Input: dimensioned drawing with shaded views. Units: mm. Origin: part minimum x, y, z. Give positions to 0.01 mm unless a question says otherwise; leave off trailing zeros. Write each loop counter-clockwise with the first axis right and the second up, starting at its lowest first coordinate (ties: lowest second). Pieces come first, ordered by that corner, then holes. Notation, with made-up numbers: (-14, 6) -> (45, 6) arc R11 ccw to (45, 18) -> close; hole circle Ø2 at (37.5, 21.5). An arc over 180 degrees is marked (long way). Return JSON: item names as keys, results as strings. Group by question number.
Item 1: Section B-B, the plane y = 72. Return loops of the section in (x, z).
Item 2: Section A-A, the plane x = 63.5. Return loops of the section in (y, z).
Item 3: Section C-C, the plane z = 3. Count the separate pieces of the cut face and the enclosed holes in it.
Item 4: Pin query (flat end, axial travel): P1, Ø1.9, axis at x = 32, z = 4, coming from the +Y side; P2, Ø3, axis at x = 124.5, z = 4.5, coming from the +Y side; P3, Ø3, axis at y = 92, z = 2, coming from the +X side. Return the tip coordinate at first contact, or that it passes through.
Item 5: Line query: line 1 (Y direction, x = 6, z = 1); line 2 (X direction, y = 86.5, z = 3.25); line 3 (X direction, y = 19, z = 1.75). Output: solid intervals per line, ascending. Write a range as [from, to].
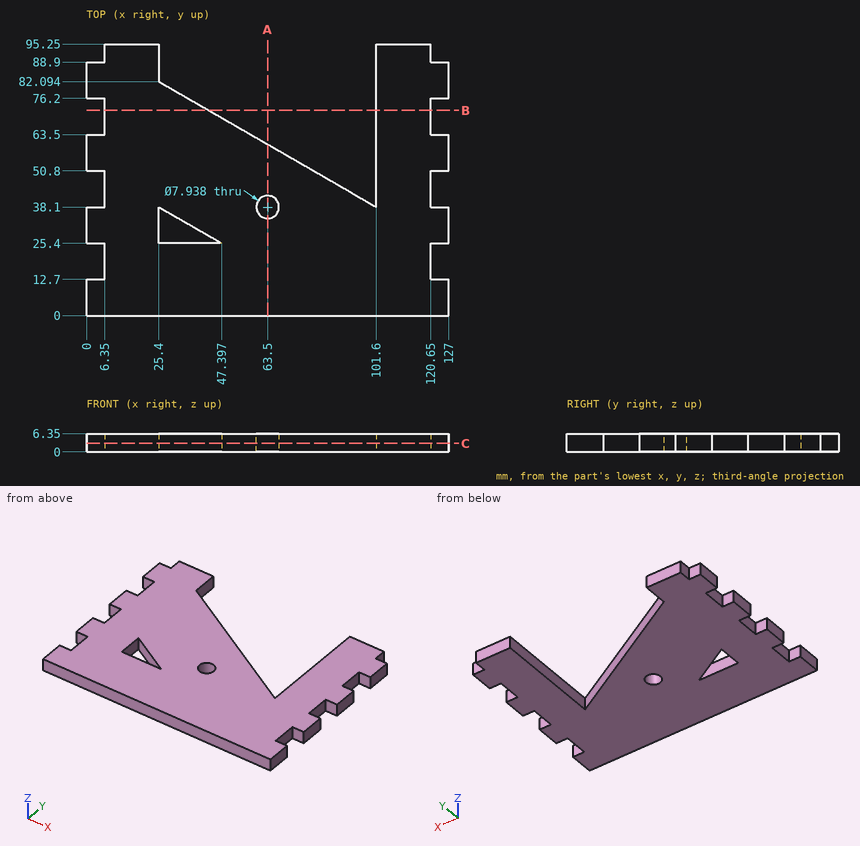
Answer below:
{
 "1": {"outline": "(6.35, 0) -> (42.88, 0) -> (42.88, 6.35) -> (6.35, 6.35) -> close; (101.6, 0) -> (120.65, 0) -> (120.65, 6.35) -> (101.6, 6.35) -> close"},
 "2": {"outline": "(0, 0) -> (34.13, 0) -> (34.13, 6.35) -> (0, 6.35) -> close; (42.07, 0) -> (60.1, 0) -> (60.1, 6.35) -> (42.07, 6.35) -> close"},
 "3": {"separate pieces": "1", "enclosed holes": "2"},
 "4": {"P1": "stops at y = 78.83", "P2": "stops at y = 88.9", "P3": "stops at x = 120.65"},
 "5": {"line 1": "y = [0, 12.7], [25.4, 38.1], [50.8, 63.5], [76.2, 88.9]", "line 2": "x = [0, 25.4], [101.6, 127]", "line 3": "x = [6.35, 120.65]"}
}
